Autodesk Inventor part; units mm, degrees
ref_plane "YZ Plane" through (0, 0, 0) normal (1, 0, 0) x (0, 1, 0)
ref_plane "XZ Plane" through (0, 0, 0) normal (0, 1, 0) x (-1, 0, 0)
ref_plane "XY Plane" through (0, 0, 0) normal (0, 0, 1) x (1, 0, 0)
sketch "Sketch1" plane through (0, 0, 0) normal (0, 1, 0) x (-1, 0, 0)
  line L0 (0, 0) -> (-20, 0)
  line L1 (-20, 0) -> (-20, -20)
  line L2 (-20, -20) -> (0, -20)
  line L3 (0, -20) -> (0, 0)
  point P0 (-10, -10)
  point P1 (-20, -10)
  point P2 (-10, -20)
  dimension "d0" = 20
  dimension "d1" = 20
extrude "Extrusion1" add sketch "Sketch1" against normal blind 15
hole "Hole1" at (10, 0, -10) direction (0, -1, 0) diameter 3.4036 end through all counterbore diameter 6.5024 counterbore depth 2.9972
fillet "Fillet1" radius 1 8 edges at (20, -7.5, 0) (10, 0, 0) (20, 0, -10) (10, 0, -20) (0, 0, -10) (20, -7.5, -20) (0, -7.5, -20) (0, -7.5, 0)
properties part number "Stop Block"
Check sheet for the modelled part. Datum: model origin and axes. Units: mm. A direction names the side the tool comes from. Round coordinates to 2 decimals unless told otherwise and drop trailing zeros. Loops run counter-clockwise (first coordinate to the right, second up) from the corner with the lowest first, then second, coordinate; pieces in that order, holes last. Notation, with made-up numbers: (5, -13) -> (9, -13) arc R14 ccw to (9, 5) -> close; hole circle Ø6 at (87.25, -27). An arc over 180 degrees is marked (long way). Answer in a Markdown table with one row per item.
Q1. Go/stop test with a flat-tipped pin: P1, Ø5, axis at x = 10, z = -10, coming from the +Y side. Record where the tip stops, or that it passes through.
Data:
| item | result |
|---|---|
| P1 | stops at y = -3 |
Q2. Sectioned sample at A-A on x = 10. Enter the section's corners in (y, z).
Data:
| item | result |
|---|---|
| outline | (-15, -20) -> (-1, -20) arc R1 ccw to (0, -19) -> (0, -13.25) -> (-3, -13.25) -> (-3, -11.7) -> (-15, -11.7) -> close; (-15, -8.3) -> (-3, -8.3) -> (-3, -6.75) -> (0, -6.75) -> (0, -1) arc R1 ccw to (-1, 0) -> (-15, 0) -> close |
Q3. Release check for a two-part mould opening along Z. For faces 1 (the face through (11.036, -9.083, -11.35)), 2 (the face through (0.285, -8.098, -19.699)), 3 (the face through (10, -8, 0)), 4 (the face through (13.174, -1.52, -10.705)) record: released by +Z, released by -Z, zero draft, split by the parting line, or undercut.
Data:
| item | result |
|---|---|
| face 1 | undercut |
| face 2 | released by -Z |
| face 3 | released by +Z |
| face 4 | undercut |
Q4. Sectioned sample at B-B on z = -10. Enter the section's corners in (x, y), then the cut area to 3 significant figures.
Data:
| item | result |
|---|---|
| outline | (0, -15) -> (8.3, -15) -> (8.3, -3) -> (6.75, -3) -> (6.75, 0) -> (1, 0) arc R1 ccw to (0, -1) -> close; (11.7, -15) -> (20, -15) -> (20, -1) arc R1 ccw to (19, 0) -> (13.25, 0) -> (13.25, -3) -> (11.7, -3) -> close |
| area | 239 mm^2 |
Q5. Thickness scan on L1, parallel to X at y = -1.75, z = -10; L2, parallel to Z at x = 10, y = -2.35; L3, parallel to Z at x = 10, y = -5.25. Record the ranges inside material, lowest first.
Data:
| item | result |
|---|---|
| L1 | x = 0 to 6.75, 13.25 to 20 |
| L2 | z = -20 to -13.25, -6.75 to 0 |
| L3 | z = -20 to -11.7, -8.3 to 0 |
Q6. Sectioned sample at C-C on y = -6.75. Enter the section's corners in (x, z), then the cut area to 3 significant figures.
Data:
| item | result |
|---|---|
| outline | (0, -19) arc R1 ccw to (1, -20) -> (19, -20) arc R1 ccw to (20, -19) -> (20, -1) arc R1 ccw to (19, 0) -> (1, 0) arc R1 ccw to (0, -1) -> close; hole circle Ø3.4 at (10, -10) |
| area | 390 mm^2 |
Q7. Set-up check for faces 5 (the face through (11.4, -2.997, -8.6)), 6 (the face through (0.301, -8.098, -0.285)): record each of +Z, -Z, +X, -X, +Y, -Y from which the full face is reachable in a straight line by a thin tool's end or side.
Data:
| item | result |
|---|---|
| face 5 | +Y |
| face 6 | +Z, -X, +Y, -Y |
